Drawing for the job (mm, zero at the part's lowest x, y, z). A direction names the side the tool comes from. Coordinates: 2 decimals unless noted, no trailing zeros. Write each loop counter-clockwise with the first axis right and the second up, starting at its lowest first coordinate (ties: lowest second). Pieces come first, ordered by that corner, then holes. Notation, with made-up numbers: M 65.5,79 L 102.5,79 A21 ccw 102.5,108 Z; hole C 36.5,-37.5 d6. An arc over 180 degrees is marked long. Put each result on its own line as item: value. Start each with the question number.
Q1. Drill centre lines: line 1 along Y through (x, z) = (8.5, 5.25); line 2 along Y through (x, z) = (10.75, 24); line 3 along X through (y, z) = (41.5, 18.5). Where is each one in solid material? Low to high.
Q2. Drop a flat-ended pin along its axis: pin 1 (12 mm diameter, centred on x = 23, z = 21.5, fed in from +Y). Give the stop position or say it passes through.
Q3. Cut at A-A (z = 15). Write the cut outline in (x, y).
Q4. Which spindle directions (+Z, -Z, +X, -X, +Y, -Y) get a long thin tool onto all of the face, cutting with end or side? Do the marked faces 1 and 2. Say none if no direction does.
Q5. Cut at B-B (x = 15). Write the cut outline in (y, z), then the cut area to 3 significant figures.
Q6. Cut at C-C (y = 46). Write the cut outline in (x, z).
Q7. Cut at D-D (z = 23). Write the cut outline in (x, y).
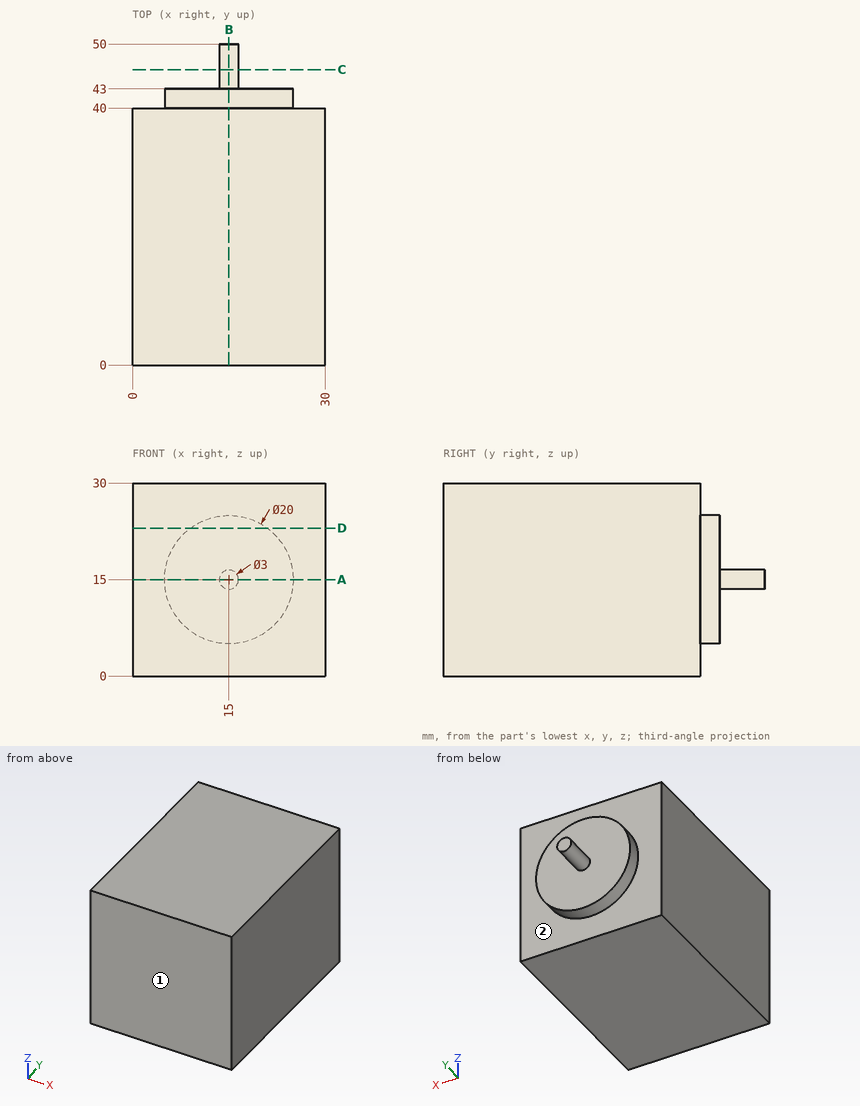
Computed values:
1. line 1: 0 to 40
1. line 2: 0 to 43
1. line 3: 5.63 to 24.37
2. pin 1: y = 43
3. outline: M 0,0 L 30,0 L 30,40 L 25,40 L 25,43 L 16.5,43 L 16.5,50 L 13.5,50 L 13.5,43 L 5,43 L 5,40 L 0,40 Z
4. face 1: +Z, -Z, +X, -X, -Y
4. face 2: +Y
5. outline: M 0,0 L 40,0 L 40,5 L 43,5 L 43,13.5 L 50,13.5 L 50,16.5 L 43,16.5 L 43,25 L 40,25 L 40,30 L 0,30 Z
5. area: 1,280 mm2
6. outline: C 15,15 d3
7. outline: M 0,0 L 30,0 L 30,40 L 21,40 L 21,43 L 9,43 L 9,40 L 0,40 Z
